from build123d import *

# Parameters (mm, degrees)
BOX038_W     = 92
BOX038_H     = 92
BOX038_DEPTH = 24
BOX034_W     = 92
BOX034_H     = 92
BOX034_DEPTH = 24
BOX036_W     = 92
BOX036_H     = 92
BOX036_DEPTH = 24
BOX037_W     = 92
BOX037_H     = 92
BOX037_DEPTH = 24
BOX035_W     = 92
BOX035_H     = 92
BOX035_DEPTH = 24
BOX032_W     = 92
BOX032_H     = 92
BOX032_DEPTH = 24
BOX030_W     = 320
BOX030_H     = 210
BOX030_DEPTH = 2
BOX039_W     = 335
BOX039_H     = 220
BOX039_DEPTH = 4
BOX031_W     = 10
BOX031_H     = 210
BOX031_DEPTH = 7
BOX028_W     = 340
BOX028_H     = 10
BOX028_DEPTH = 7
BOX027_W     = 10
BOX027_H     = 210
BOX027_DEPTH = 15
BOX033_W     = 10
BOX033_H     = 210
BOX033_DEPTH = 15
BOX026_W     = 340
BOX026_H     = 10
BOX026_DEPTH = 15
BOX025_W     = 340
BOX025_H     = 10
BOX025_DEPTH = 15
BOX029_W     = 10
BOX029_H     = 210
BOX029_DEPTH = 7


with BuildPart() as obj1:
    # Box038 → Box038 (new body)
    with BuildSketch(Plane(origin=(14, 124, 0), x_dir=(1, 0, 0), z_dir=(0, 0, 1))):
        with Locations((46, 46)):
            Rectangle(BOX038_W, BOX038_H)
    extrude(amount=BOX038_DEPTH)


with BuildPart() as obj2:
    # Box034 → Box034 (new body)
    with BuildSketch(Plane(origin=(124, 124, 0), x_dir=(1, 0, 0), z_dir=(0, 0, 1))):
        with Locations((46, 46)):
            Rectangle(BOX034_W, BOX034_H)
    extrude(amount=BOX034_DEPTH)


with BuildPart() as obj3:
    # Box036 → Box036 (new body)
    with BuildSketch(Plane(origin=(234, 124, 0), x_dir=(1, 0, 0), z_dir=(0, 0, 1))):
        with Locations((46, 46)):
            Rectangle(BOX036_W, BOX036_H)
    extrude(amount=BOX036_DEPTH)


with BuildPart() as obj4:
    # Box037 → Box037 (new body)
    with BuildSketch(Plane(origin=(234, 15, 0), x_dir=(1, 0, 0), z_dir=(0, 0, 1))):
        with Locations((46, 46)):
            Rectangle(BOX037_W, BOX037_H)
    extrude(amount=BOX037_DEPTH)


with BuildPart() as obj5:
    # Box035 → Box035 (new body)
    with BuildSketch(Plane(origin=(124, 15, 0), x_dir=(1, 0, 0), z_dir=(0, 0, 1))):
        with Locations((46, 46)):
            Rectangle(BOX035_W, BOX035_H)
    extrude(amount=BOX035_DEPTH)


with BuildPart() as obj6:
    # Box032 → Box032 (new body)
    with BuildSketch(Plane(origin=(14, 14, 0), x_dir=(1, 0, 0), z_dir=(0, 0, 1))):
        with Locations((46, 46)):
            Rectangle(BOX032_W, BOX032_H)
    extrude(amount=BOX032_DEPTH)


with BuildPart() as obj7:
    # Box030 → Box030 (new body)
    with BuildSketch(Plane(origin=(10, 10, 8), x_dir=(1, 0, 0), z_dir=(0, 0, 1))):
        with Locations((160, 105)):
            Rectangle(BOX030_W, BOX030_H)
    extrude(amount=BOX030_DEPTH)


with BuildPart() as obj8:
    # Box039 → Box039 (new body)
    with BuildSketch(Plane(origin=(5, 5, 4), x_dir=(1, 0, 0), z_dir=(0, 0, 1))):
        with Locations((167.5, 110)):
            Rectangle(BOX039_W, BOX039_H)
    extrude(amount=BOX039_DEPTH)


with BuildPart() as obj9:
    # Box031 → Box031 (new body)
    with BuildSketch(Plane(origin=(220, 10, 8), x_dir=(1, 0, 0), z_dir=(0, 0, 1))):
        with Locations((5, 105)):
            Rectangle(BOX031_W, BOX031_H)
    extrude(amount=BOX031_DEPTH)


with BuildPart() as base007:
    # Box028 → Box028 (new body)
    with BuildSketch(Plane(origin=(0, 110, 8), x_dir=(1, 0, 0), z_dir=(0, 0, 1))):
        with Locations((170, 5)):
            Rectangle(BOX028_W, BOX028_H)
    extrude(amount=BOX028_DEPTH)


with BuildPart() as obj10:
    # Box027 → Box027 (new body)
    with BuildSketch(Plane(origin=(330, 10, 0), x_dir=(1, 0, 0), z_dir=(0, 0, 1))):
        with Locations((5, 105)):
            Rectangle(BOX027_W, BOX027_H)
    extrude(amount=BOX027_DEPTH)


with BuildPart() as obj11:
    # Box033 → Box033 (new body)
    with BuildSketch(Plane(origin=(0, 10, 0), x_dir=(1, 0, 0), z_dir=(0, 0, 1))):
        with Locations((5, 105)):
            Rectangle(BOX033_W, BOX033_H)
    extrude(amount=BOX033_DEPTH)


with BuildPart() as base006:
    # Box026 → Box026 (new body)
    with BuildSketch(Plane(origin=(0, 220, 0), x_dir=(1, 0, 0), z_dir=(0, 0, 1))):
        with Locations((170, 5)):
            Rectangle(BOX026_W, BOX026_H)
    extrude(amount=BOX026_DEPTH)


with BuildPart() as base005:
    # Box025 → Box025 (new body)
    with BuildSketch(Plane.XY):
        with Locations((170, 5)):
            Rectangle(BOX025_W, BOX025_H)
    extrude(amount=BOX025_DEPTH)


with BuildPart() as baseoriginal:
    # Box029 → Box029 (new body)
    with BuildSketch(Plane(origin=(110, 10, 8), x_dir=(1, 0, 0), z_dir=(0, 0, 1))):
        with Locations((5, 105)):
            Rectangle(BOX029_W, BOX029_H)
    extrude(amount=BOX029_DEPTH)

    # Fusion003: union obj9, base007, obj10, obj11, base006, base005
    add(obj9.part)
    add(base007.part)
    add(obj10.part)
    add(obj11.part)
    add(base006.part)
    add(base005.part)

    # Cut012: cut obj8
    add(obj8.part, mode=Mode.SUBTRACT)

    # Fusion002: union obj7
    add(obj7.part)

    # Cut008: cut obj6
    add(obj6.part, mode=Mode.SUBTRACT)

    # Cut009: cut obj5
    add(obj5.part, mode=Mode.SUBTRACT)

    # Cut014: cut obj4
    add(obj4.part, mode=Mode.SUBTRACT)

    # Cut010: cut obj3
    add(obj3.part, mode=Mode.SUBTRACT)

    # Cut011: cut obj2
    add(obj2.part, mode=Mode.SUBTRACT)

    # Cut013: cut obj1
    add(obj1.part, mode=Mode.SUBTRACT)


with BuildPart() as baseoriginal_1:
    # Cut013 placement: moved
    add(baseoriginal.part.moved(Location((353, 251, 0))))


solid = baseoriginal_1.part
Can you work these out from the model? Positions are in its coordinate system, mm. A direction names the side the tool comes from. Coordinates: 2 decimals unless noted, no trailing zeros. Write each loop counter-clockwise with the first axis right and the second up, starting at its lowest first coordinate (ties: lowest second). Pieces come first, ordered by that corner, then holes. Notation, with made-up numbers: (20, 10) -> (24, 10) arc R19 cw to (24, 32) -> close; hole circle Ø7 at (-30, 52.5). An arc over 180 degrees is marked (long way). Write item = value, one per line.
(1) Imagine slicing it at A-A (y = 367). Please give me the cut outline in (x, z).
Verdict:
outline = (353, 0) -> (363, 0) -> (363, 4) -> (358, 4) -> (358, 8) -> (693, 8) -> (693, 15) -> (353, 15) -> close; (683, 0) -> (693, 0) -> (693, 4) -> (683, 4) -> close
(2) Imagine slicing it at B-B (x = 416). Please give me the cut outline in (y, z).
Verdict:
outline = (251, 0) -> (261, 0) -> (261, 4) -> (256, 4) -> (256, 8) -> (265, 8) -> (265, 10) -> (261, 10) -> (261, 15) -> (251, 15) -> close; (357, 8) -> (375, 8) -> (375, 10) -> (371, 10) -> (371, 15) -> (361, 15) -> (361, 10) -> (357, 10) -> close; (467, 8) -> (476, 8) -> (476, 4) -> (471, 4) -> (471, 0) -> (481, 0) -> (481, 15) -> (471, 15) -> (471, 10) -> (467, 10) -> close
(3) If I drill on probe 1 along Y at (x, z) = (608, 14); probe 2 along X at (y, z) = (460, 12.5); probe 3 along Y at (x, z) = (372.5, 9.75), over which ranges is the centre line in solid material (lowest first)?
Verdict:
probe_1 = 251 to 261, 361 to 371, 471 to 481
probe_2 = 353 to 363, 463 to 473, 573 to 583, 683 to 693
probe_3 = 251 to 265, 357 to 375, 467 to 481
(4) Imagine slicing it at C-C (y = 280). State how many separate pieces and enclosed holes the cut face has, and give its area (3 significant figures).
Verdict:
separate_pieces = 5
enclosed_holes = 0
area = 428 mm^2
(5) Thinking about a two-plate mould opening in Y: for faces 1 (the face through (521, 251, 7)), 2 (the face through (519, 373, 10)), 3 (the face through (521, 481, 7)), which applies, +Y half, -Y half, draft (parallel to the pull), parting line (faces both ways), or undercut?
Verdict:
face_1 = -Y half
face_2 = undercut
face_3 = +Y half
(6) On a 3-axis mill with a long thin cutter (end or side, diameter ignored), from which of +Z, -Z, +X, -X, +Y, -Y can I reach the whole of each face in a straight line? I mean faces 4 (the face through (510, 367, 15)), 5 (the face through (409, 263, 10)), 6 (the face through (574, 472, 4)). Say none if no direction works.
Verdict:
face_4 = +Z, +X, -X, +Y, -Y
face_5 = +Z
face_6 = +X
